Geometry check sheet. Reference: the model listing, model coordinates, mm. A direction names the side the tool comes from. Coordinates: 2 decimals unless noted, no trailing zeros. Order: outer loops, then holes, each group sorted by start corner. A loop starts at its lowest first (then second) coordinate and runs counter-clockwise, first axis right, second up. Notation, with made-up numbers: (41.5, 82.25) - (45.5, 82.25) arc R13 cw to (45.5, 93.25) - close; hole circle Ø5 at (-3, 81). An arc over 180 degrees is marked (long way). Return JSON: item names as keys, results as strings. Group by question number.
Item 1: Section check A-A on y = 8.75. Enter the section's corners in (x, z).
Item 2: Section check D-D on z = -88.5. Enter the section's corners in (x, y).
Item 3: Draft check along X on faces 4 (the flat face through (-5, 13, -39)), 5 (the flat face through (164, 7, -76)), 6 (the flat face through (76, 0, -20)), 7 (the flat face through (76, 25, -107)). Enter one of: pulls with the +X half, pulls with the -X half, needs draft (parallel to the pull), parting line crosses it, or undercut.
Item 4: Scan lines: probe 1 along Y at (x, z) = (74.5, -99.5); probe 2 along X at (y, z) = (12.75, -63); probe 3 along X at (y, z) = (2.25, -67). Record each from-to range of solid material in increasing order.
Item 5: Tool access check on faces 1 (the flat face through (161, 3, 11)), 2 (the flat face through (156, 7, 5)), 3 (the flat face through (0, 10, -63)). Record the directions out of +Z, -Z, +X, -X, +Y, -Y that give a thin tool (end or side, any length) a straight path to the whole face; none if there is none.
Item 6: Section check C-C on z = 7. Enter the section's corners in (x, y).
Item 7: Gauge pin test, flat ends, axial feed: pin 1 (1.5 mm diameter, centred on x = 68, z = -60, fed in from +Y); pin 2 (5.5 mm diameter, centred on x = 160.5, y = 5, fed in from +Z); pin 3 (4 mm diameter, centred on x = 18.5, y = 20, fed in from +Z). Record the tip position at first contact, or that the pin passes through.
Item 8: Section check B-B on x = 23. Enter the section's corners in (y, z), then the cut area to 3 significant figures.
from build123d import *

# Parameters (mm, degrees)
SKETCH1_W           = 164
SKETCH1_H           = 94
BOSS_EXTRUDE1_DEPTH = 5
BOSS_EXTRUDE2_DEPTH = 5
SKETCH2_W           = 164
SKETCH2_H           = 30
BOSS_EXTRUDE3_DEPTH = 5
SKETCH3_W           = 5
SKETCH3_H           = 94
BOSS_EXTRUDE4_DEPTH = 10
SKETCH4_W           = 5
SKETCH4_H           = 100
BOSS_EXTRUDE5_DEPTH = 16
SKETCH5_W           = 5
SKETCH5_H           = 5
CUT_EXTRUDE1_DEPTH  = 4
BOSS_EXTRUDE6_DEPTH = 40
BOSS_EXTRUDE7_DEPTH = 45
SKETCH9_W           = 164
SKETCH9_H           = 5
BOSS_EXTRUDE8_DEPTH = 10


with BuildPart() as part:
    # Sketch1 → Boss-Extrude1 (new body)
    with BuildSketch(Plane(origin=(0, 0, 0), x_dir=(1, 0, 0), z_dir=(0, 1, 0))):
        with Locations((77, 42)):
            Rectangle(SKETCH1_W, SKETCH1_H)
    extrude(amount=-BOSS_EXTRUDE1_DEPTH)

    # Sketch1<3> → Boss-Extrude2 (add)
    with BuildSketch(Plane(origin=(0, 0, 0), x_dir=(1, 0, 0), z_dir=(0, 1, 0))):
        Polygon((0, -5), (0, 0), (0, 84), (154, 84), (154, 0), (154, -5), (159, -5), (159, 89), (-5, 89), (-5, -5), align=None)
    extrude(amount=BOSS_EXTRUDE2_DEPTH)

    # Sketch2 → Boss-Extrude3 (add)
    with BuildSketch(Plane(origin=(0, -5, 0), x_dir=(-1, 0, 0), z_dir=(0, -1, 0))):
        with Locations((-77, -20)):
            Rectangle(SKETCH2_W, SKETCH2_H)
    extrude(amount=-BOSS_EXTRUDE3_DEPTH)

    # Sketch3 → Boss-Extrude4 (add)
    with BuildSketch(Plane(origin=(0, 5, 0), x_dir=(1, 0, 0), z_dir=(0, 1, 0))):
        with Locations((-2.5, 42)):
            Rectangle(SKETCH3_W, SKETCH3_H)
        with Locations((156.5, 42)):
            Rectangle(SKETCH3_W, SKETCH3_H)
    extrude(amount=BOSS_EXTRUDE4_DEPTH)

    # Sketch4 → Boss-Extrude5 (add)
    with BuildSketch(Plane.XZ.offset(5)):
        with Locations((-7.5, -39)):
            Rectangle(SKETCH4_W, SKETCH4_H)
        with Locations((161.5, -39)):
            Rectangle(SKETCH4_W, SKETCH4_H)
    extrude(amount=-BOSS_EXTRUDE5_DEPTH)

    # Sketch5 → Cut-Extrude1 (cut)
    with BuildSketch(Plane(origin=(0, 15, 0), x_dir=(1, 0, 0), z_dir=(0, 1, 0))):
        with Locations((-2.5, 86.5)):
            Rectangle(SKETCH5_W, SKETCH5_H)
        with Locations((156.5, 86.5)):
            Rectangle(SKETCH5_W, SKETCH5_H)
    extrude(amount=-CUT_EXTRUDE1_DEPTH, mode=Mode.SUBTRACT)

    # Sketch6 → Boss-Extrude6 (add)
    with BuildSketch(Plane(origin=(0, 0, -89), x_dir=(-1, 0, 0), z_dir=(0, 0, -1))):
        Polygon((10, -5), (10, 11), (0, 11), (0, 5), (-154, 5), (-154, 11), (-164, 11), (-164, -5), align=None)
    extrude(amount=BOSS_EXTRUDE6_DEPTH)

    # Sketch8 → Boss-Extrude7 (add)
    with BuildSketch(Plane(origin=(0, 0, -129), x_dir=(-1, 0, 0), z_dir=(0, 0, -1))):
        Polygon((-164, 11), (-154, 11), (-154, 20), (0, 20), (0, 11), (10, 11), (10, 25), (-164, 25), align=None)
    extrude(amount=-BOSS_EXTRUDE7_DEPTH)

    # Sketch9 → Boss-Extrude8 (add)
    with BuildSketch(Plane.XY.offset(35)):
        with Locations((77, -2.5)):
            Rectangle(SKETCH9_W, SKETCH9_H)
    extrude(amount=BOSS_EXTRUDE8_DEPTH)


solid = part.part
Computed:
{
 "1": {"outline": "(-10, -129) - (0, -129) - (0, 5) - (-5, 5) - (-5, 11) - (-10, 11) - close; (154, -129) - (164, -129) - (164, 11) - (159, 11) - (159, 5) - (154, 5) - close"},
 "2": {"outline": "(-10, -5) - (164, -5) - (164, 25) - (-10, 25) - close; hole (0, 5) - (154, 5) - (154, 20) - (0, 20) - close"},
 "3": {"face 4": "pulls with the -X half", "face 5": "pulls with the +X half", "face 6": "undercut", "face 7": "needs draft"},
 "4": {"probe 1": "y = -5 to 5, 20 to 25", "probe 2": "x = -5 to 0, 154 to 159", "probe 3": "x = -10 to 0, 154 to 164"},
 "5": {"face 1": "+Z, +X, +Y, -Y", "face 2": "+Z, +Y", "face 3": "+Z"},
 "6": {"outline": "(-10, -5) - (164, -5) - (164, 11) - (159, 11) - (159, 0) - (-5, 0) - (-5, 11) - (-10, 11) - close"},
 "7": {"pin 1": "stops at y = 0", "pin 2": "stops at z = 11", "pin 3": "stops at z = -84"},
 "8": {"outline": "(-5, -129) - (5, -129) - (5, -84) - (0, -84) - (0, 45) - (-5, 45) - close; (20, -129) - (25, -129) - (25, -84) - (20, -84) - close", "area": "1,320 mm²"}
}
